For this review, take the finished solid that the model builds, in its own axes (mm). Face numbers are marked on the shaded views. Give positions to 0.01 mm unless a question says otherwise; leave off trailing zeros. Order: outer loops, then holes, each group sorted by start corner. A loop starts at its lowest first (then second) coordinate and runs counter-clockwise, first axis right, second up.
Item 1: Consider section B-B (z = 0). Give the boundary of the cut face in (x, y).
Item 2: For probe 1 along Z at (x, y) = (0, -4.25); probe 2 along Z at (x, y) = (-0.25, -0.5); probe 3 along Z at (x, y) = (-1.75, -3), list the stretches that pass through material, from the lowest coordinate up.
Item 3: Consider section D-D (x = -3.5). Give the boundary of the cut face in (y, z).
Item 4: Consider section A-A (y = 0). Give the boundary of the cut face in (x, z).
Item 5: The part is to be moulded in two halves that separate along Z. For the marked faces 1, 2, 3 and 4, say which applies: released by +Z, released by -Z, zero draft, split by the parting line, or undercut.
Item 6: Consider section C-C (x = 0). Give the boundary of the cut face in (y, z), plus the area to 3 significant figures.
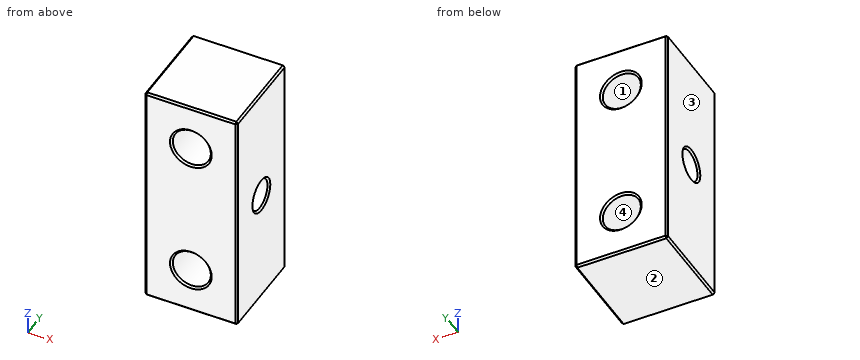
```python
from build123d import *

# Parameters (mm, degrees)
SKETCH_1_W              = 10
SKETCH_1_H              = 10
EXTRUDE_1_DEPTH         = 12.5
HOLE_WIZARD_M4_1_D      = 3.3
HOLE_WIZARD_4_1_4_1_1_D = 4.1
CHAMFER_1_SIZE          = 0.2


with BuildPart() as part:
    # 草图1 → 凸台-拉伸1 (new, symmetric)
    with BuildSketch(Plane.XY):
        Rectangle(SKETCH_1_W, SKETCH_1_H)
    extrude(amount=EXTRUDE_1_DEPTH, both=True)

    # M4 螺纹孔1 (through all)
    with Locations(Plane(origin=(5, 0, 0), x_dir=(0, 0, -1), z_dir=(1, 0, 0))):
        with Locations((0, 0)):
            Hole(HOLE_WIZARD_M4_1_D / 2)

    # Ø4.1 (4.1) 直径孔1 (through all)
    with Locations(Plane(origin=(0, 5, 0), x_dir=(1, 0, 0), z_dir=(0, 1, 0))):
        with Locations((0, -7.5), (0, 7.5)):
            Hole(HOLE_WIZARD_4_1_4_1_1_D / 2)

    # 倒角1
    chamfer_1_edges = [part.edges().sort_by_distance(p)[0] for p in [
        (-5, 0, 12.5),
        (5, 0, -1.65),
        (-5, 0, -1.65),
        (0, -5, 12.5),
        (2.05, 5, -7.5),
        (2.05, -5, -7.5),
        (2.05, 5, 7.5),
        (2.05, -5, 7.5),
        (5, 0, 12.5),
        (0, -5, -12.5),
        (-5, 0, -12.5),
        (0, 5, -12.5),
        (5, 0, -12.5),
        (5, -5, 0),
        (-5, -5, 0),
        (-5, 5, 0),
        (5, 5, 0),
        (0, 5, 12.5),
    ]]
    chamfer(chamfer_1_edges, length=CHAMFER_1_SIZE)


solid = part.part
```
Resolved:
1. outline: (-5, -4.8) - (-4.8, -5) - (4.8, -5) - (5, -4.8) - (5, -1.85) - (4.8, -1.65) - (-4.8, -1.65) - (-5, -1.85) - close; (-5, 1.85) - (-4.8, 1.65) - (4.8, 1.65) - (5, 1.85) - (5, 4.8) - (4.8, 5) - (-4.8, 5) - (-5, 4.8) - close
2. probe 1: z = -12.5 to -9.55, -5.45 to 5.45, 9.55 to 12.5
2. probe 2: z = -12.5 to -9.53, -5.47 to -1.57, 1.57 to 5.47, 9.53 to 12.5
2. probe 3: z = -12.5 to -8.57, -6.43 to 6.43, 8.57 to 12.5
3. outline: (-5, -12.3) - (-4.8, -12.5) - (4.8, -12.5) - (5, -12.3) - (5, 12.3) - (4.8, 12.5) - (-4.8, 12.5) - (-5, 12.3) - close; hole circle Ø3.3 at (0, 0)
4. outline: (-5, -12.3) - (-4.8, -12.5) - (4.8, -12.5) - (5, -12.3) - (5, -1.85) - (4.8, -1.65) - (-4.8, -1.65) - (-5, -1.85) - close; (-5, 1.85) - (-4.8, 1.65) - (4.8, 1.65) - (5, 1.85) - (5, 12.3) - (4.8, 12.5) - (-4.8, 12.5) - (-5, 12.3) - close; hole circle Ø4.1 at (0, -7.5); hole circle Ø4.1 at (0, 7.5)
5. face 1: undercut
5. face 2: released by -Z
5. face 3: zero draft
5. face 4: undercut
6. outline: (-5, -12.3) - (-4.8, -12.5) - (4.8, -12.5) - (5, -12.3) - (5, -9.75) - (4.8, -9.55) - (-4.8, -9.55) - (-5, -9.75) - close; (-5, -5.25) - (-4.8, -5.45) - (4.8, -5.45) - (5, -5.25) - (5, 5.25) - (4.8, 5.45) - (-4.8, 5.45) - (-5, 5.25) - close; (-5, 9.75) - (-4.8, 9.55) - (4.8, 9.55) - (5, 9.75) - (5, 12.3) - (4.8, 12.5) - (-4.8, 12.5) - (-5, 12.3) - close; hole circle Ø3.3 at (0, 0)
6. area: 159 mm2
